CAD build for the part. Positions are in the model's coordinates, mm. A direction names the side the tool comes from. Round coordinates to 2 decimals unless told otherwise and drop trailing zeros. Loops run counter-clockwise (first coordinate to the right, second up) from the corner with the lowest first, then second, coordinate; pieces in that order, holes last. Notation, with made-up numbers: M -14.5,-22.5 L 18.5,-22.5 A30 cw 18.5,3.5 Z; hole C 26.5,-8.75 d9. An arc over 180 degrees is marked long. Use a Markdown table: item, result. Add a question column.
(1) Flat gauge pins, fed straight in: P1, Ø3, axis at x = 0, y = 8.5, coming from the +Z side; P2, Ø4, axis at y = 8, z = 2, coming from the +X side; P3, Ø1, axis at x = 3, z = 3.5, coming from the -Y side. Where does each tip first touch, or does it go through?
(2) Band-saw the part on D-D, the plane x = 2.75. Write the cut outline in (y, z), and give its area (3 significant figures).
(3) Which spindle directions (+Z, -Z, +X, -X, +Y, -Y) get a long thin tool onto all of the face, cutting with end or side? Do faces 1 (the face through (2.028, 1.87, -3.448)), 2 (the face through (-0.54, 11.09, 2.44)). Say none if no direction does.
(4) Band-saw the part on B-B, the plane x = -2.25. Write the cut outline in (y, z), and give its area (3 significant figures).
(5) Wall check: L1, parallel to Z at x = 0, y = 15.25; L2, parallel to Z at x = 3.5, y = 3; L3, parallel to X at y = 2, z = 2.75. Give the ranges that are in metal, low to high.
(6) Band-saw the part on C-C, the plane y = 13. Write the cut outline in (x, z).
(7) Band-saw the part on A-A, the plane z = 0. Write the cut outline in (x, y).
from build123d import *

# Parameters (mm, degrees)
EXTRUDE_1_DEPTH = 3.2
SKETCH_2_R      = 2.5
EXTRUDE_2_DEPTH = 16
CHAMFER_1_SIZE  = 1
CHAMFER_1_SIZE2 = 0.577350269


with BuildPart() as part:
    # Эскиз1 → Бобышка-Вытянуть1 (new body)
    with BuildSketch(Plane(origin=(0, 0, 0), x_dir=(1, 0, 0), z_dir=(0, 1, 0))):
        Polygon((4, -2.309401077), (4, 2.309401077), (0, 4.618802154), (-4, 2.309401077), (-4, -2.309401077), (0, -4.618802154), align=None)
    extrude(amount=EXTRUDE_1_DEPTH)

    # Эскиз2 → Бобышка-Вытянуть2 (add)
    with BuildSketch(Plane(origin=(0, 3.2, 0), x_dir=(1, 0, 0), z_dir=(0, 1, 0))):
        Circle(SKETCH_2_R)
    extrude(amount=EXTRUDE_2_DEPTH)

    # Фаска1
    chamfer_1_edges = [part.edges().sort_by_distance(p)[0] for p in [
        (-2, 0, 3.464101615),
        (-4, 0, 0),
        (-2, 0, -3.464101615),
        (2, 0, -3.464101615),
        (4, 0, 0),
        (2, 0, 3.464101615),
    ]]
    chamfer_1_side = [part.faces().sort_by_distance(p)[0] for p in [
        (0, 0, 0),
    ]]
    chamfer(chamfer_1_edges, length=CHAMFER_1_SIZE, length2=CHAMFER_1_SIZE2, reference=chamfer_1_side[0])


solid = part.part
Return value:
| question | item | result |
|---|---|---|
| 1 | P1 | z = 2.5 |
| 1 | P2 | x = 2.5 |
| 1 | P3 | through |
| 2 | outline | M 0,-1.88 L 0.58,-3.03 L 3.2,-3.03 L 3.2,3.03 L 0.58,3.03 L 0,1.88 Z |
| 2 | area | 18.7 mm^2 |
| 3 | face 1 | -Z, +X, +Y, -Y |
| 3 | face 2 | +Y |
| 4 | outline | M 0,-2.17 L 0.58,-3.32 L 3.2,-3.32 L 3.2,-1.09 L 19.2,-1.09 L 19.2,1.09 L 3.2,1.09 L 3.2,3.32 L 0.58,3.32 L 0,2.17 Z |
| 4 | area | 55.5 mm^2 |
| 5 | L1 | -2.5 to 2.5 |
| 5 | L2 | -2.6 to 2.6 |
| 5 | L3 | -3.24 to 3.24 |
| 6 | outline | C 0,0 d5 |
| 7 | outline | M -4,0.58 L -3,0 L 3,0 L 4,0.58 L 4,3.2 L 2.5,3.2 L 2.5,19.2 L -2.5,19.2 L -2.5,3.2 L -4,3.2 Z |
